```python
from build123d import *

# Parameters (mm, degrees)
F0_W     = 230
F0_H     = 114
F1_DEPTH = 76
F3_W     = 38
F3_H     = 20
F4_DEPTH = 230.001
F6_W     = 38
F6_H     = 38
F7_DEPTH = 114.001


with BuildPart() as f1:
    # F0 (on Front) → F1 (new body)
    with BuildSketch(Plane.XZ):
        Rectangle(F0_W, F0_H)
    extrude(amount=F1_DEPTH)

    # F3 (on offset) → F4 (cut, through all)
    with BuildSketch(Plane.YZ.offset(115)):
        with Locations((-19, 47)):
            Rectangle(F3_W, F3_H)
    extrude(amount=-F4_DEPTH, mode=Mode.SUBTRACT)

    # F6 (on offset) → F7 (cut, through all)
    with BuildSketch(Plane.XY.offset(57)):
        with Locations((-96, -57)):
            Rectangle(F6_W, F6_H)
        with Locations((96, -57)):
            Rectangle(F6_W, F6_H)
    extrude(amount=-F7_DEPTH, mode=Mode.SUBTRACT)


solid = f1.part
```
Here's how the part is built. I have some questions about the finished solid (model axes, mm). A direction names the side the tool comes from. Coordinates: 2 decimals unless noted, no trailing zeros. Loops run counter-clockwise (first coordinate to the right, second up) from the corner with the lowest first, then second, coordinate; pieces in that order, holes last. Notation, with made-up numbers: (58.5, -39) - (94.5, -39) arc R22 cw to (94.5, -10) - close; hole circle Ø7 at (16, 72.5). An arc over 180 degrees is marked (long way). Answer as CSV lines item,"result".
Q1. If I drill on L1, parallel to Y at x = 79, z = 29.5; L2, parallel to Z at x = -25, y = -31.5; L3, parallel to X at y = -56.5, z = -13.5, over which ranges is the centre line in solid material (lowest first)? Write a range as [from, to].
Response:
L1,"[-38, 0]"
L2,"[-57, 37]"
L3,"[-77, 77]"
Q2. If we section it at B-B, the plane x = 23.5: Write out the boundary of the cut face in (y, z), and give its area (3 significant figures).
Response:
outline,"(-76, -57) - (0, -57) - (0, 37) - (-38, 37) - (-38, 57) - (-76, 57) - close"
area,"7,900 mm2"
Q3. For pin 1 (8 mm diameter, centred on x = -77.5, z = 40.5, fed in from +Y); pin 2 (19 mm diameter, centred on x = -96, z = 8, fed in from -Y); pin 3 (19 mm diameter, centred on x = -12.5, y = -15.5, fed in from +Z); pin 4 (10 mm diameter, centred on x = 28, z = 42.5, fed in from +Y), each with a flat end and sliding along its axis, tell me the tip position at first contact or that it passes through.
Response:
pin 1,"y = 0"
pin 2,"y = -38"
pin 3,"z = 37"
pin 4,"y = -38"
Q4. If we section it at D-D, the plane y = -35: Write out the boundary of the cut face in (x, z).
Response:
outline,"(-115, -57) - (115, -57) - (115, 37) - (-115, 37) - close"
Q5. For faces 1 (the face through (1, -38, 47)), 2 (the face through (96, -38, -9)), 3 (the face through (-77, -57, 1)), which set-ups out of +Z, -Z, +X, -X, +Y, -Y let a thin tool reach every point of the face, with its end or its side?
Response:
face 1,"+Z, +X, -X, +Y"
face 2,"+Z, -Z, +X, -Y"
face 3,"+Z, -Z, -X, -Y"
Q6. If we section it at C-C, the plane y = -62.5: Write out the boundary of the cut face in (x, z), and give its area (3 significant figures).
Response:
outline,"(-77, -57) - (77, -57) - (77, 57) - (-77, 57) - close"
area,"17,600 mm2"
Q7. If we section it at A-A, the plane z = 10.5: Write out the boundary of the cut face in (x, y).
Response:
outline,"(-115, -38) - (-77, -38) - (-77, -76) - (77, -76) - (77, -38) - (115, -38) - (115, 0) - (-115, 0) - close"
